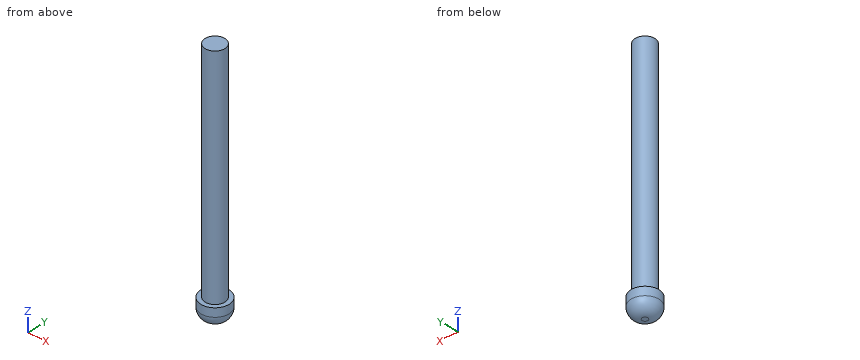
```python
from build123d import *

# Parameters (mm, degrees)
F0_R     = 1.75
F1_DEPTH = 40
F0_R_2   = 2.5
F2_DEPTH = 3.5
F3_R     = 2


with BuildPart() as f1:
    # F0 (on Top) → F1 (new body)
    with BuildSketch(Plane.XY):
        Circle(F0_R)
    extrude(amount=F1_DEPTH)

    # F0 (on Top) → F2 (join)
    with BuildSketch(Plane.XY):
        Circle(F0_R_2)
        Circle(F0_R, mode=Mode.SUBTRACT)
        Circle(F0_R)
    extrude(amount=-F2_DEPTH)

    # F3
    f3_edges = [f1.edges().sort_by_distance(p)[0] for p in [
        (-2.5, 0, -3.5),
    ]]
    fillet(f3_edges, radius=F3_R)


solid = f1.part
```
Geometry check sheet. Reference: the model listing, model coordinates, mm. Coordinates: 2 decimals unless noted, no trailing zeros. Order: outer loops, then holes, each group sorted by start corner. A loop starts at its lowest first (then second) coordinate and runs counter-clockwise, first axis right, second up. Notation, with made-up numbers: (53.5, 48) - (79.5, 48) arc R22 ccw to (79.5, 84) - close; hole circle Ø5 at (-39, -17.5). An arc over 180 degrees is marked (long way). Use one line per item in the form item = value.
1. Scan lines: line 1 (Y direction, x = 0.1, z = 5); line 2 (Z direction, x = -0.55, y = -1.1); line 3 (Z direction, x = 1.55, y = 0.25). Record each from-to range of solid material in increasing order.
Here are the results:
line_1 = -1.75 to 1.75
line_2 = -3.36 to 40
line_3 = -3.19 to 40
2. Gauge pin test, flat ends, axial feed: pin 1 (1.5 mm diameter, centred on x = -1.5, y = -0.5, fed in from -Z); pin 2 (2 mm diameter, centred on x = 0.5, z = 24, fed in from -Y); pin 3 (1 mm diameter, centred on x = 1.5, z = 20, fed in from -Y). Record the tip position at first contact, or that the pin passes through.
Here are the results:
pin_1 = -3.47
pin_2 = -1.75
pin_3 = -1.44
3. Section check A-A (z = 37). Record the boundary of the cut face in (x, y).
Here are the results:
outline = circle Ø3.5 at (0, 0)
